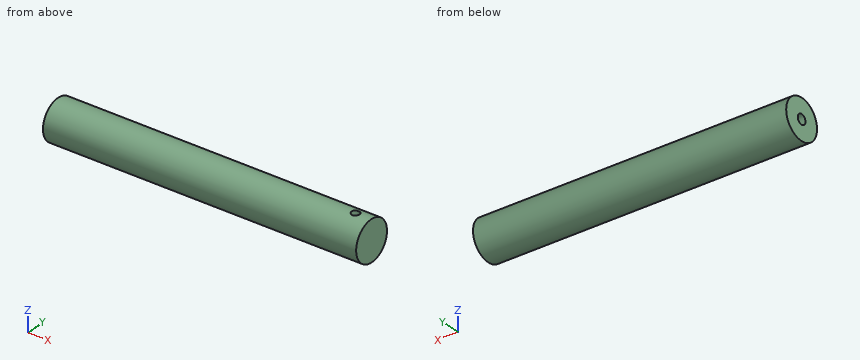
Autodesk Inventor part; units mm, degrees
ref_plane "作業平面1" through (0, 0, 5) normal (0, 0, 1) x (1, 0, 0)
ref_plane "YZ Plane" through (0, 0, 0) normal (1, 0, 0) x (0, 1, 0)
ref_plane "XZ Plane" through (0, 0, 0) normal (0, 1, 0) x (-1, 0, 0)
sketch "スケッチ1" plane through (0, 0, 0) normal (1, 0, 0) x (0, 1, 0)
  circle A0 centre (0, 0) radius 5
  dimension "d0" = 10
extrude "押し出し1" add sketch "スケッチ1" along normal blind 79
sketch "スケッチ2" plane through (0, 0, 0) normal (-1, 0, 0) x (0, 0, 1)
  circle A0 centre (0, 0) radius 1.25
  dimension "d3" = 2.5
extrude "押し出し2" cut sketch "スケッチ2" against normal blind 5
ref_plane "作業平面1" through (0, 0, 5) normal (0, 0, 1) x (1, 0, 0)
sketch "スケッチ3" plane through (0, 0, 5) normal (0, 0, 1) x (1, 0, 0)
  line L0 (79, -5) -> (79, 5)
  point P0 (0, 0)
  point P1 (75, 0)
  dimension "d6" = 4
hole "穴1" at (75, 0, 5) direction (0, 0, -1) diameter 2 depth 5 tip angle 118
properties part number "belt_liner_v5_shaft_2" material "アルミニウム 6061"
Can you work these out from the model? Positions are in its coordinate system, mm. Coordinates: 2 decimals unless noted, no trailing zeros. Loops run counter-clockwise (first coordinate to the right, second up) from the corner with the lowest first, then second, coordinate; pieces in that order, holes last. Notation, with made-up numbers: (56.5, 68.5) -> (65.5, 68.5) arc R25 ccw to (65.5, 106.5) -> close; hole circle Ø3 at (-23, 32.25). An arc over 180 degrees is marked (long way). Put each result on its own line as item: value. Start each with the question number.
Q1. I want a section at D-D (y = 3.25). Write out the boundary of the cut face in (x, z), plus the area to 3 significant figures.
Q2. I want a section at B-B (z = 3.25). Write out the boundary of the cut face in (x, y), plus the area to 3 significant figures.
Q3. I'm going to push flat-ended pins straight in: P1, Ø1, axis at x = 67.5, z = -1, coming from the +Y side; P2, Ø3, axis at x = 53.5, y = 2, coming from the +Z side; P3, Ø2, axis at y = 0, z = 0, coming from the -X side. Where does each tip first touch, or does it pass through?
Q4. I want a section at C-C (x = 6). Write out the boundary of the cut face in (y, z).
Q5. I want a section at A-A (z = -4). Write out the boundary of the cut face in (x, y).
Q6. If I drill on line 1 (X direction, y = 0, z = 1.2); line 2 (Y direction, x = 75, z = 2.55); line 3 (Y direction, x = 75, z = 1.1), over which ranges is the centre line in solid material (lowest first)? Write a range as [from, to].
Taken from the geometry:
1. outline: (0, -3.8) -> (79, -3.8) -> (79, 3.8) -> (0, 3.8) -> close
1. area: 600 mm2
2. outline: (0, -3.8) -> (79, -3.8) -> (79, 3.8) -> (0, 3.8) -> close; hole circle Ø2 at (75, 0)
2. area: 597 mm2
3. P1: stops at y = 4.97
3. P2: stops at z = 4.97
3. P3: stops at x = 5
4. outline: circle Ø10 at (0, 0)
5. outline: (0, -3) -> (79, -3) -> (79, 3) -> (0, 3) -> close
6. line 1: x = [5, 74], [76, 79]
6. line 2: y = [-4.3, -1], [1, 4.3]
6. line 3: y = [-4.88, -1], [1, 4.88]
